The figure shows three views and two pictorial views of one solid part (mm, origin at its lowest corner). Answer the questions. Coordinates: 2 decimals unless noted, no trailing zeros. Loops run counter-clockwise (first coordinate to the right, second up) from the corner with the lowest first, then second, coordinate; pieces in that order, holes last. Notation, with made-up numbers: M 55.5,36 L 79.5,36 A25 ccw 79.5,59 Z; hole C 40.25,62 d1. An arc over 180 degrees is marked long. Return JSON: item names as keys, results as strings. Group by question number.
1. Section C-C (x = 3.5) is taken. Write down the section's boundary in (y, z).
2. Section D-D (x = 1.2) is taken. Write down the section's boundary in (y, z).
3. Section A-A (z = 11) is taken. Write down the section's boundary in (x, y), then the cut area to 3 significant figures.
4. Section B-B (x = 2.1) is taken. Write down the section's boundary in (y, z).
5. Straight lines are drawn through the part: L1, parallel to Y at x = 2, z = 11.25 (1 decimal); L2, parallel to X at y = 1.55, z = 12.25 (1 decimal); L3, parallel to Y at x = 1.7, z = 5 (1 decimal). For each, find the intervals that lie inside material, in ascending order. Write a range as from..to.
6. Given P1, Ø2, axis at y = 3.5, z = 12, coming from the -X side; P2, Ø1, axis at x = 2.5, z = 10.5, coming from the -Y side, each flat-ended and moving along its own axis, determine where each tip first touches the part or whether it passes through.
7. The mould has two halves that part along Y. Classify the marked faces 1, 2, 3 and 4: pulls with the +Y half, pulls with the -Y half, needs draft (parallel to the pull), parting line crosses it, or undercut.
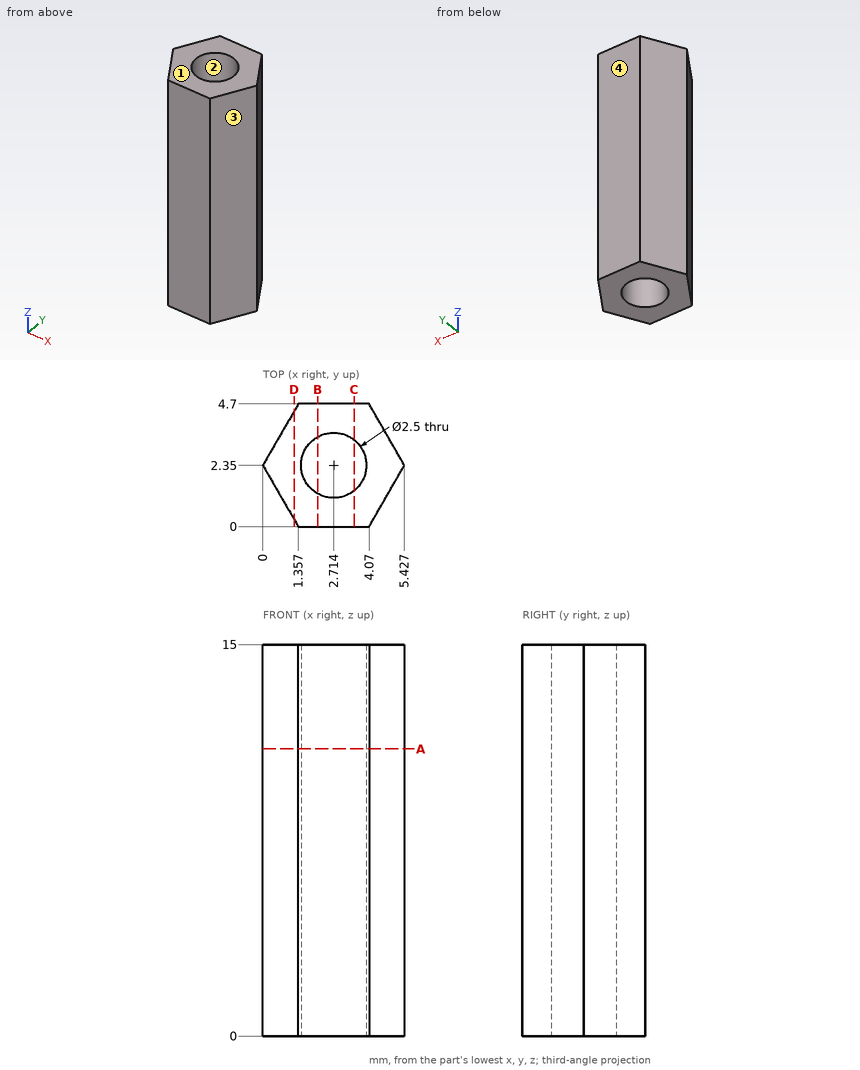
Worked out:
{
 "1": {"outline": "M 0,0 L 1.38,0 L 1.38,15 L 0,15 Z; M 3.32,0 L 4.7,0 L 4.7,15 L 3.32,15 Z"},
 "2": {"outline": "M 0.27,0 L 4.43,0 L 4.43,15 L 0.27,15 Z"},
 "3": {"outline": "M 0,2.35 L 1.36,0 L 4.07,0 L 5.43,2.35 L 4.07,4.7 L 1.36,4.7 Z; hole C 2.71,2.35 d2.5", "area": "14.2 mm^2"},
 "4": {"outline": "M 0,0 L 1.26,0 L 1.26,15 L 0,15 Z; M 3.44,0 L 4.7,0 L 4.7,15 L 3.44,15 Z"},
 "5": {"L1": "0..1.3, 3.4..4.7", "L2": "0.5..1.8, 3.7..5", "L3": "0..1.6, 3.1..4.7"},
 "6": {"P1": "x = 0.09", "P2": "y = 0"},
 "7": {"face 1": "needs draft", "face 2": "undercut", "face 3": "pulls with the -Y half", "face 4": "pulls with the +Y half"}
}
